```python
from build123d import *

# Parameters (mm, degrees)
BOSS_SWITCHMAIN_DEPTH                          = 3
SKETCH1_W                                      = 4
SKETCH1_H                                      = 3.5
BOSS_FLANGE_WIDTH_DEPTH                        = 5
BOSS_FLANGE_HEIGHT_REACH                       = 38.958
SKETCH2_W                                      = 4
SKETCH2_H                                      = 2
SKETCH2_W_2                                    = 8
SKETCH2_H_2                                    = 2.024994097
CUT_UP_TO_DOWN_DERAILLEUR_CLEARANCE_REACH      = 27.678
SKETCH10_W                                     = 2.453096586
SKETCH10_H                                     = 3
SKETCH17_W                                     = 12.1675
SKETCH17_H                                     = 4
BOSS_FLANGE_SUPPORT_DEPTH                      = 14.475002167
TAP_DRILL_FOR_M2X0_4_TAP1_D                    = 1.6
M2_CLEARANCE_HOLE2_D                           = 2.4
M2_CLEARANCE_HOLE2_DEPTH                       = 15
M2_CLEARANCE_HOLE2_TIP                         = 0.721032743
CUT_UP_TO_DOWN_CANTILEVER_SLOPE_REACH          = 32.725
CUT_DOWN_TO_UP_DERAILLEUR_CLEARANCE_DEPTH      = 34.178566414
CUT_DOWN_TO_UP_DERAILLEUR_CLEARANCE_DEPTH_BACK = 34.178566414
CHAMFER_FLANGE_SUPPORT_SIZE                    = 1.5
CHAMFER_FLANGE_SUPPORT_2_SIZE                  = 1
CHAMFER_FLANGE_SUPPORT_3_SIZE                  = 1
SKETCH18_W                                     = 1.5
SKETCH18_H                                     = 1.577350269
CUT_DOWN_TO_UP_DERAILLEUR_CLEARANCE_2_DEPTH    = 1


with BuildPart() as part:
    # Sketch-SwitchBossUp → Boss-SwitchMain (new body)
    with BuildSketch(Plane.XY):
        with BuildLine():
            Line((6.540476927, 22.165014537), (6.540476927, 25.000549624))
            Line((6.540476927, 25.000549624), (8.540476927, 25.000549624))
            Line((8.540476927, 25.000549624), (8.540476927, 20.473554675))
            Line((8.540476927, 20.473554675), (2.463355023, 19.450530066))
            Line((2.463355023, 19.450530066), (3.620297651, 12.577888564))
            Line((3.620297651, 12.577888564), (4.256080915, 12.944958203))
            Line((4.256080915, 12.944958203), (4.256080915, 14.944958203))
            Line((4.256080915, 14.944958203), (3.581073513, 15.334673908))
            Line((3.581073513, 15.334673908), (3.581073513, 18.834673908))
            Line((3.581073513, 18.834673908), (6.857327822, 18.834673908))
            Line((6.857327822, 18.834673908), (15.309115797, 18.834673908))
            Line((15.309115797, 18.834673908), (15.309115797, -1.165326092))
            Line((15.309115797, -1.165326092), (5.040476927, -1.165326092))
            Line((5.040476927, -1.165326092), (3.040476927, -1.165326092))
            Line((3.040476927, -1.165326092), (3.040476927, 0.859668005))
            Line((3.040476927, 0.859668005), (4.040476927, 1.437018274))
            Line((4.040476927, 1.437018274), (4.040476927, 3.937018274))
            Line((4.040476927, 3.937018274), (2.83114552, 4.326720436))
            Line((2.83114552, 4.326720436), (2.83114552, 4.826720436))
            Line((2.83114552, 4.826720436), (3.58114552, 4.826720436))
            Line((3.58114552, 4.826720436), (4.256138119, 5.216427595))
            Line((4.256138119, 5.216427595), (4.256138119, 7.216427595))
            Line((4.256138119, 7.216427595), (3.581130717, 7.6061433))
            Line((3.581130717, 7.6061433), (2.9061262, 7.216422599))
            Line((2.9061262, 7.216422599), (0.971281627, 7.216422599))
            Line((0.971281627, 7.216422599), (0.971281627, 9.019692757))
            Line((0.971281627, 9.019692757), (1.971281627, 9.019692757))
            Line((1.971281627, 9.019692757), (2.646271341, 9.40939825))
            Line((2.646271341, 9.40939825), (2.646271341, 11.40939825))
            Line((2.646271341, 11.40939825), (0.897326855, 12.41915182))
            Line((0.897326855, 12.41915182), (0.545466745, 12.771663724))
            Line((0.545466745, 12.771663724), (-0.372784255, 18.226393961))
            ThreePointArc((-0.372784255, 18.226393961), (-0.209313172, 18.996084896), (0.435897335, 19.446473985))
            Line((0.435897335, 19.446473985), (-0.46073685, 24.772792819))
            ThreePointArc((-0.46073685, 24.772792819), (-2.387846783, 25.912534906), (-3.038018253, 28.054973186))
            ThreePointArc((-3.038018253, 28.054973186), (-2.23296648, 28.745546602), (-1.542393064, 27.940494829))
            ThreePointArc((-1.542393064, 27.940494829), (0.129544452, 26.234339128), (1.59980805, 28.11706781))
            ThreePointArc((1.59980805, 28.11706781), (2.195840434, 28.994419163), (3.073191787, 28.398386779))
            ThreePointArc((3.073191787, 28.398386779), (2.830256228, 26.496543155), (1.511513111, 25.104801997))
            Line((1.511513111, 25.104801997), (2.131345845, 21.422780026))
            Line((2.131345845, 21.422780026), (6.540476927, 22.165014537))
        make_face()
        Polygon((5.581091201, 12.555245643), (5.581100766, 11.263016278), (3.971265023, 11.263016278), (3.97126394, 11.79911022), (3.296271341, 11.409403061), (3.296271341, 9.409403061), (3.971278743, 9.019687356), (3.971278743, 9.409408058), (5.815189335, 10.763016278), (6.627976927, 9.860324206), (6.627976927, 8.210536506), (5.581127833, 7.606137899), (4.906138119, 7.216432406), (4.906138119, 5.216432406), (5.58114552, 4.826716701), (6.33114552, 4.826716701), (6.33114552, 4.326716701), (5.040476927, 3.937018274), (5.040476927, 1.437018274), (6.040476927, 0.859668005), (9.127976927, 0.859668005), (10.437466736, 2.169157813), (10.437466736, 14.025180364), (9.127976927, 15.334670172), (5.581073513, 15.334670172), (4.906080915, 14.944963014), (4.906080915, 12.944963014), align=None, mode=Mode.SUBTRACT)
    extrude(amount=BOSS_SWITCHMAIN_DEPTH)

    # Sketch1 → Boss-Flange Width (add)
    with BuildSketch(Plane(origin=(0, 0, 0), x_dir=(-1, 0, 0), z_dir=(0, 0, -1))):
        Polygon((-7.581073513, -1.165326092), (0.412170615, -1.165326092), (0.412170615, 0.859668005), (-3.040476927, 0.859668005), (-4.040476927, 1.437018274), (-5.040476927, 1.437018274), (-6.040476927, 0.859668005), (-7.581073513, 0.859668005), align=None)
        with Locations((-5.581073513, 17.084673908)):
            Rectangle(SKETCH1_W, SKETCH1_H)
    extrude(amount=BOSS_FLANGE_WIDTH_DEPTH)

    # Sketch2 → Boss-Flange Height (add, up to next)
    with BuildSketch(Plane(origin=(-7.039523073, 0, 0), x_dir=(0, 0, -1), z_dir=(1, 0, 0)), mode=Mode.PRIVATE) as boss_flange_height_sk1:
        with Locations((3, 16.334673908)):
            Rectangle(SKETCH2_W, SKETCH2_H)
    boss_flange_height_tool1 = extrude(boss_flange_height_sk1.sketch, amount=BOSS_FLANGE_HEIGHT_REACH, mode=Mode.PRIVATE) - part.part
    # Sketch2 → Boss-Flange Height (add, up to next)
    with BuildSketch(Plane(origin=(-7.039523073, 0, 0), x_dir=(0, 0, -1), z_dir=(1, 0, 0)), mode=Mode.PRIVATE) as boss_flange_height_sk2:
        with Locations((1, -0.152829044)):
            Rectangle(SKETCH2_W_2, SKETCH2_H_2)
    boss_flange_height_tool2 = extrude(boss_flange_height_sk2.sketch, amount=BOSS_FLANGE_HEIGHT_REACH, mode=Mode.PRIVATE) - part.part
    add(boss_flange_height_tool1.solids().sort_by_distance((-7.039523, 16.334674, -3))[0])
    add(boss_flange_height_tool2.solids().sort_by_distance((-7.039523, -0.152829, -1))[0])

    # Sketch10 → Cut-Up-To-Down Derailleur Clearance (cut, up to next)
    with BuildSketch(Plane(origin=(0, 18.834673908, 0), x_dir=(1, 0, 0), z_dir=(0, 1, 0)), mode=Mode.PRIVATE) as cut_up_to_down_derailleur_clearance_sk1:
        with Locations((6.35452522, 3.5)):
            Rectangle(SKETCH10_W, SKETCH10_H)
    cut_up_to_down_derailleur_clearance_tool1 = extrude(cut_up_to_down_derailleur_clearance_sk1.sketch, amount=-CUT_UP_TO_DOWN_DERAILLEUR_CLEARANCE_REACH, mode=Mode.PRIVATE) & part.part
    add(cut_up_to_down_derailleur_clearance_tool1.solids().sort_by_distance((6.354525, 18.834674, -3.5))[0], mode=Mode.SUBTRACT)


with BuildPart() as boss_flange_support_tool:
    # Sketch17 → Boss-Flange Support (new body)
    with BuildSketch(Plane.XZ.offset(-15.334670172)):
        with Locations((-0.955773073, -3)):
            Rectangle(SKETCH17_W, SKETCH17_H)
    extrude(amount=BOSS_FLANGE_SUPPORT_DEPTH)


with BuildPart() as part_1:
    add(part.part)


with BuildPart() as part_2:
    # Boss-Flange Support: joined with boss_flange_support_tool
    add(part_1.part.fuse(boss_flange_support_tool.part, tol=0.00001))

    # Tap Drill for M2x0.4 Tap1 (through all)
    with Locations(Plane(origin=(0, -1.165326092, 0), x_dir=(-1, 0, 0), z_dir=(0, -1, 0))):
        with Locations((4.039523073, 3), (-0.581073513, 3)):
            Hole(TAP_DRILL_FOR_M2X0_4_TAP1_D / 2)

    # M2 Clearance Hole2
    with Locations(Plane.XZ.offset(1.165326092)):
        with Locations((-4.039523073, -3), (0.581073513, -3)):
            Hole(M2_CLEARANCE_HOLE2_D / 2, depth=M2_CLEARANCE_HOLE2_DEPTH)
            with Locations((0, 0, -(M2_CLEARANCE_HOLE2_DEPTH + M2_CLEARANCE_HOLE2_TIP / 2))):  # 118° drill point
                Cone(0, M2_CLEARANCE_HOLE2_D / 2, M2_CLEARANCE_HOLE2_TIP, mode=Mode.SUBTRACT)

    # Sketch12 → Cut-Up-to-Down Cantilever Slope (cut, up to next)
    with BuildSketch(Plane(origin=(0, 25.000549624, 0), x_dir=(1, 0, 0), z_dir=(0, 1, 0)), mode=Mode.PRIVATE) as cut_up_to_down_cantilever_slope_sk1:
        Polygon((6.540476927, 0), (8.540476927, -3), (8.540476927, 0), align=None)
    cut_up_to_down_cantilever_slope_tool1 = extrude(cut_up_to_down_cantilever_slope_sk1.sketch, amount=-CUT_UP_TO_DOWN_CANTILEVER_SLOPE_REACH, mode=Mode.PRIVATE) & part_2.part
    add(cut_up_to_down_cantilever_slope_tool1.solids().sort_by_distance((7.87381, 25.00055, 1))[0], mode=Mode.SUBTRACT)

    # Sketch16 → Cut-Down-to-Up Derailleur Clearance (cut, two sides: drawn at the far end of the back side and taken through both)
    with BuildSketch(Plane(origin=(0, 0, 0), x_dir=(-1, 0, 0), z_dir=(0, 0, -1)).offset(-CUT_DOWN_TO_UP_DERAILLEUR_CLEARANCE_DEPTH_BACK)):
        Polygon((-6.627976927, 18.834673908), (-15.309115797, 18.834673908), (-15.309115797, -1.165326092), (-6.627976927, -1.165326092), (-6.627976927, 5.203794929), (-8.003689255, 5.203794929), (-8.003689255, 12.048417413), (-6.627976927, 12.048417413), align=None)
    extrude(amount=CUT_DOWN_TO_UP_DERAILLEUR_CLEARANCE_DEPTH + CUT_DOWN_TO_UP_DERAILLEUR_CLEARANCE_DEPTH_BACK, mode=Mode.SUBTRACT)

    # Chamfer-Flange Support
    chamfer_flange_support_edges = [part_2.edges().sort_by_distance(p)[0] for p in [
        (3.581073513, 17.334673908, -3),
    ]]
    chamfer(chamfer_flange_support_edges, length=CHAMFER_FLANGE_SUPPORT_SIZE - 0.0001)  # a hair under: the kernel refuses the full size

    # Chamfer-Flange Support 2
    chamfer_flange_support_2_edges = [part_2.edges().sort_by_distance(p)[0] for p in [
        (5.127976927, 17.084673908, -2),
        (5.127976927, 15.334670172, -1.5),
    ]]
    chamfer(chamfer_flange_support_2_edges, length=CHAMFER_FLANGE_SUPPORT_2_SIZE)

    # Chamfer-Flange Support 3
    chamfer_flange_support_3_edges = [part_2.edges().sort_by_distance(p)[0] for p in [
        (-1.999523073, 0.859668005, -1),
    ]]
    chamfer(chamfer_flange_support_3_edges, length=CHAMFER_FLANGE_SUPPORT_3_SIZE)

    # Sketch18 → Cut-Down-to-Up Derailleur Clearance 2 (cut)
    with BuildSketch(Plane(origin=(6.627976927, 0, 0), x_dir=(0, 0, -1), z_dir=(1, 0, 0))):
        with Locations((-2.25, 0.64834314)):
            Rectangle(SKETCH18_W, SKETCH18_H)
    extrude(amount=-CUT_DOWN_TO_UP_DERAILLEUR_CLEARANCE_2_DEPTH, mode=Mode.SUBTRACT)


solid = part_2.part
```
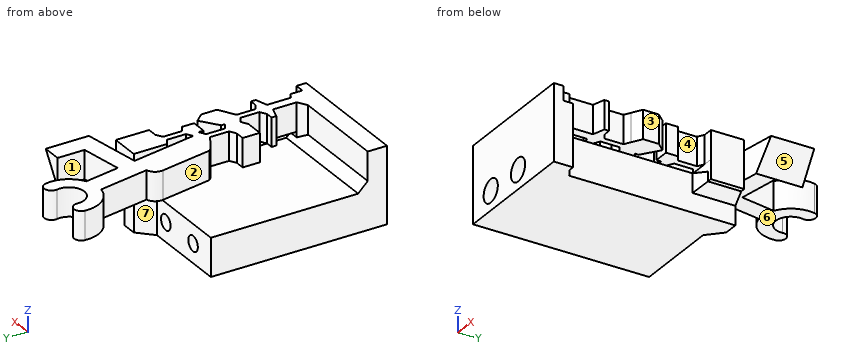
Build history of the part. All positions in model axes, mm. Face numbers are marked on the shaded views. A direction names the side the tool comes from. Give positions to 0.01 mm unless a question says otherwise; leave off trailing zeros. Order: outer loops, then holes, each group sorted by start corner. A loop starts at its lowest first (then second) coordinate and runs counter-clockwise, first axis right, second up. Notation, with made-up numbers: M -8.75,-1.5 L 38.25,-1.5 A30 cw 38.25,28.5 Z; hole C -37.5,84.25 d8. An arc over 180 degrees is marked long. Return JSON: item names as keys, results as strings.
Q1. 3-axis set-ups, long thin cutter, end or side, ignore diameter. For the marked faces 1, 2, 3 and 4: which of +Z, -Z, +X, -X, +Y, -Y reach the whole face in a straight line?
Answer list:
{"face 1": "+Z, -Z, +Y", "face 2": "+Z, -X", "face 3": "+Z, -Z, +X, -Y", "face 4": "+Z, +X"}
Q2. Band-saw the part on A-A (y = 27). Give the cut face in (x, z), then the cut area to 3 significant figures.
Answer list:
{"outline": "M -2.94,0 L -1.32,0 L -1.32,3 L -2.94,3 Z; M 1.4,0 L 3.02,0 L 3.02,3 L 1.4,3 Z", "area": "9.70 mm^2"}
Q3. Flat gauge pins, fed straight in: pin 1 (4 mm diameter, centred on x = 0.04, y = 27.82, fed in from -Z); pin 2 (1 mm diameter, centred on y = 6.5, z = 1.5, fed in from +X); pin 3 (3 mm diameter, centred on y = 23, z = 2, fed in from -X). Where does each tip first touch, or does it go through?
Answer list:
{"pin 1": "stops at z = 0", "pin 2": "stops at x = 4.91", "pin 3": "stops at x = -0.41"}
Q4. Two-plate mould, pull along Y, no slides. Class the marked faces 5, 6 and 7: pulls with the +Y half, pulls with the -Y half, needs draft (parallel to the pull), parting line crosses it, or undercut.
Answer list:
{"face 5": "needs draft", "face 6": "undercut", "face 7": "pulls with the +Y half"}
Q5. Wall check: probe 1 along X at (y, z) = (6.5, -3); probe 2 along Y at (x, z) = (6.5, 2.5); probe 3 along Y at (x, z) = (5, 2.75). Give the ranges that are in metal, low to high. Write a range as from..to.
Answer list:
{"probe 1": "x = -7.04..-5.24, -2.84..-0.62, 1.78..5.13", "probe 2": "y = -1.17..-0.14, 8.14..10, 15.33..18.83, 20.13..22.16", "probe 3": "y = -1.17..5.16, 7.27..10.16, 11.26..12.89, 15..18.83, 19.88..21.91"}
Q6. Band-saw the part on B-B (z = -2.5). Count the separate pieces of the cut face and the enclosed holes in it, then the cut area to 3 significant figures.
Answer list:
{"separate pieces": "3", "enclosed holes": "0", "area": "160 mm^2"}
